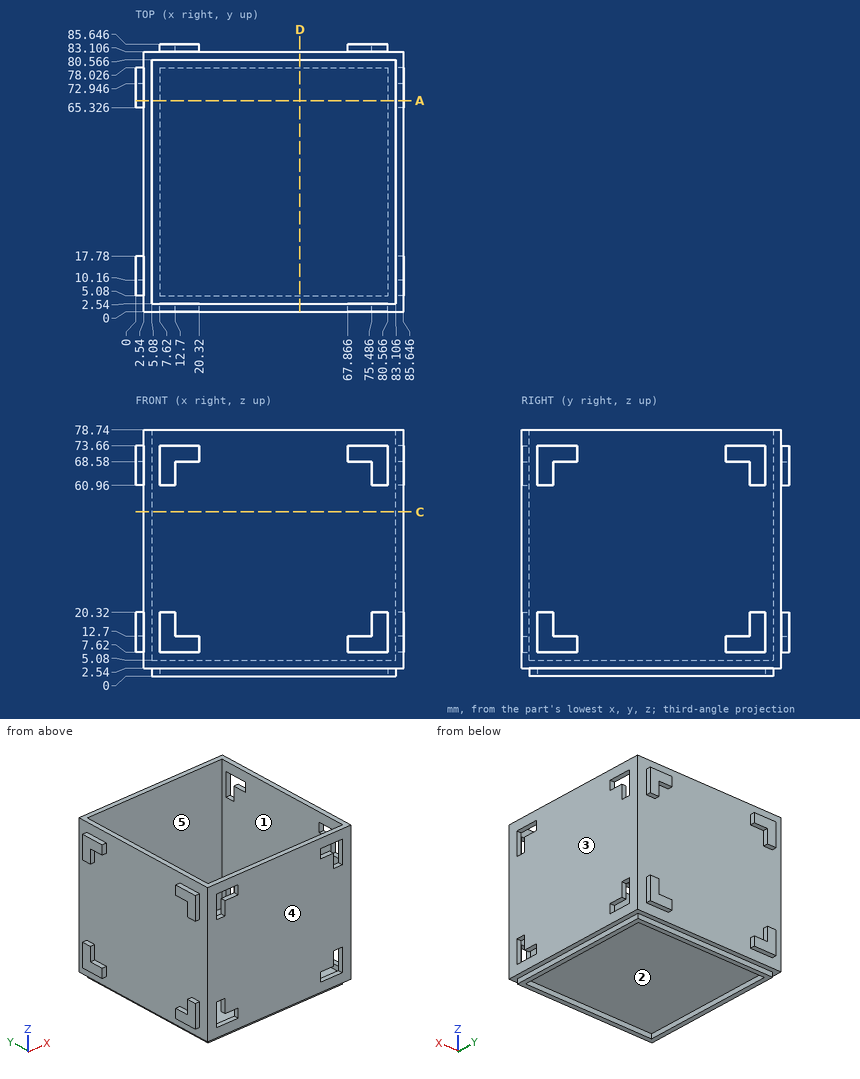
Verification items for this drawing (mm, ordinates from the low corner). A direction names the side the tool comes from. Round coordinates to 2 decimals unless told otherwise and drop trailing zeros. Order: outer loops, then holes, each group sorted by start corner. A loop starts at its lowest first (then second) coordinate and runs counter-clockwise, first axis right, second up. Notation, with made-up numbers: (13.25, -3.75) - (34.25, -3.75) arc R23 cw to (34.25, 11.25) - close; hole circle Ø4 at (71, 21). An arc over 180 degrees is marked (long way). Use CSV: the item, a comma, the result in double quotes. Start each with the question number.
1) Access from +Z, -Z, +X, -X, +Y, -Y to the whole of each face (thin tool, end or side, straight path). Record for the marked faces 1 and 2.
2) Mould release check, pull along X, two halves, no side actions. Record for the marked faces 3, 4 and 5: +X half, -X half, draft (parallel to the pull), parting line (faces both ways), or undercut.
3) Go/stop test with flat-tipped pins: P1, Ø1.3, axis at x = 84.5, y = 13, coming from the -Z side; P2, Ø1, axis at x = 53, z = 32, coming from the +Y side; P3, Ø3, axis at x = 1, y = 69.5, coming from the -Z side. Record where each tip stops, or that it passes through.
4) Section check D-D, the plane x = 52.5. Record the cut outline in (y, z).
5) Section check C-C, the plane z = 52.5. Record the cut outline in (x, y).
6) Section check A-A, the plane y = 67.5. State how many separate pieces and enclosed holes the cut face has.
7) Thickness scan on L1, parallel to Y at x = 70, z = 60.5; L2, parallel to X at y = 15, z = 59.5; L3, parallel to X at y = 82.5, z = 7. Record the ranges inside material, lowest first.
Answers:
1,face 1,"+Z"
1,face 2,"-Z"
2,face 3,"+X half"
2,face 4,"draft"
2,face 5,"undercut"
3,P1,"stops at z = 2.54"
3,P2,"stops at y = 83.11"
3,P3,"stops at z = 7.62"
4,outline,"(0, 2.54) - (2.54, 2.54) - (2.54, 0) - (5.08, 0) - (5.08, 2.54) - (78.03, 2.54) - (78.03, 0) - (80.57, 0) - (80.57, 2.54) - (83.11, 2.54) - (83.11, 78.74) - (80.57, 78.74) - (80.57, 5.08) - (2.54, 5.08) - (2.54, 78.74) - (0, 78.74) - close"
5,outline,"(2.54, 0) - (85.65, 0) - (85.65, 83.11) - (2.54, 83.11) - close; hole (5.08, 2.54) - (83.11, 2.54) - (83.11, 80.57) - (5.08, 80.57) - close"
6,separate pieces,"3"
6,enclosed holes,"0"
7,L1,"y = 0 to 2.54, 80.57 to 83.11"
7,L2,"x = 2.54 to 5.08, 83.11 to 85.65"
7,L3,"x = 2.54 to 85.65"
